from build123d import *

# Parameters (mm, degrees)
ESQUISSE1_W                                        = 11
ESQUISSE1_H                                        = 6
BOSS_EXTRU_1_DEPTH                                 = 22
DIAM_TRE_DU_PER_AGE_7_1_7_1_1_D                    = 7.1
DIAM_TRE_DU_PER_AGE_7_1_7_1_1_DEPTH                = 6
DIAM_TRE_DU_PER_AGE_8_5_8_5_1_D                    = 8.5
CHAMBRAGE_POUR_VIS_T_TE_HEXAGONALE_M21_D           = 2.5
CHAMBRAGE_POUR_VIS_T_TE_HEXAGONALE_M21_CBORE_D     = 4
CHAMBRAGE_POUR_VIS_T_TE_HEXAGONALE_M21_CBORE_DEPTH = 4.5
DIAM_TRE_DU_PER_AGE_8_0_8_1_D                      = 8
DIAM_TRE_DU_PER_AGE_8_0_8_1_DEPTH                  = 2
DIAM_TRE_DU_PER_AGE_8_0_8_1_TIP                    = 4
CHANFREIN1_SIZE                                    = 9
CHANFREIN1_SIZE2                                   = 4.785384885
ENL_V_MAT_EXTRU_1_DEPTH                            = 10


with BuildPart() as part:
    # Esquisse1 → Révolution1 (revolve)
    with BuildSketch(Plane(origin=(0, 0, 0), x_dir=(-1, 0, 0), z_dir=(0, 0, -1)), mode=Mode.PRIVATE) as r_volution1_sk:
        with Locations((-5.5, 3)):
            Rectangle(ESQUISSE1_W, ESQUISSE1_H)
    revolve(r_volution1_sk.sketch.rotate(Axis((0, 0, 0), (0, 1, 0)), 270), axis=Axis((0, 0, 0), (0, 1, 0)))

    # Esquisse2 → Boss.-Extru.1 (add)
    with BuildSketch(Plane(origin=(0, 6, 0), x_dir=(-1, 0, 0), z_dir=(0, 1, 0))):
        Polygon((-9.95156463, 2.63938656), (-3.016441782, 9.843834567), (10.088792211, -2.771484138), (3.016441782, -9.843834567), align=None)
    extrude(amount=BOSS_EXTRU_1_DEPTH)

    # Diamètre du perçage Ø7.1 (7.1)1
    with Locations(Plane(origin=(0, 28, 0), x_dir=(1, 0, 0), z_dir=(0, 1, 0))):
        with Locations((0, 0)):
            Hole(DIAM_TRE_DU_PER_AGE_7_1_7_1_1_D / 2, depth=DIAM_TRE_DU_PER_AGE_7_1_7_1_1_DEPTH)

    # Diamètre du perçage Ø8.5 (8.5)1 (through all)
    with Locations(Plane(origin=(-3.467561424, 0, 3.602224003), x_dir=(0.7204448006982934, 0, 0.6935122847843406), z_dir=(-0.6935122847843406, 0, 0.7204448006982934))):
        with Locations((-0.19047619, 17)):
            Hole(DIAM_TRE_DU_PER_AGE_8_5_8_5_1_D / 2)

    # Chambrage pour vis à tête hexagonale M21 (through all)
    with Locations(Plane(origin=(0, 6, 0), x_dir=(1, 0, 0), z_dir=(0, 1, 0))):
        with Locations((5.656854249, 5.656854249), (-5.656854249, -5.656854249)):
            CounterBoreHole(CHAMBRAGE_POUR_VIS_T_TE_HEXAGONALE_M21_D / 2, CHAMBRAGE_POUR_VIS_T_TE_HEXAGONALE_M21_CBORE_D / 2, CHAMBRAGE_POUR_VIS_T_TE_HEXAGONALE_M21_CBORE_DEPTH)

    # Diamètre du perçage Ø8.0 (8)1
    with Locations(Plane(origin=(0, 0, 0), x_dir=(-1, 0, 0), z_dir=(0, -1, 0))):
        with Locations((0, 0)):
            Hole(DIAM_TRE_DU_PER_AGE_8_0_8_1_D / 2, depth=DIAM_TRE_DU_PER_AGE_8_0_8_1_DEPTH)
            with Locations((0, 0, -(DIAM_TRE_DU_PER_AGE_8_0_8_1_DEPTH + DIAM_TRE_DU_PER_AGE_8_0_8_1_TIP / 2))):  # 90° drill point
                Cone(0, DIAM_TRE_DU_PER_AGE_8_0_8_1_D / 2, DIAM_TRE_DU_PER_AGE_8_0_8_1_TIP, mode=Mode.SUBTRACT)

    # Chanfrein1
    chanfrein1_edges = [part.edges().sort_by_distance(p)[0] for p in [
        (-6.552616997, 28, -6.307659352),
    ]]
    chanfrein1_side = [part.faces().sort_by_distance(p)[0] for p in [
        (-6.552616997, 17, -6.307659352),
    ]]
    chamfer(chanfrein1_edges, length=CHANFREIN1_SIZE, length2=CHANFREIN1_SIZE2, reference=chanfrein1_side[0])

    # Esquisse11 → Enlèv. mat.-Extru.1 (cut)
    with BuildSketch(Plane(origin=(0, 6, 0), x_dir=(1, 0, 0), z_dir=(0, 1, 0))):
        Polygon((1.20429729, -11.726353602), (11.620583405, -0.905551522), (15.545873169, -4.684101481), (5.129587053, -15.504903562), align=None)
        Polygon((0.545569668, 13.405846017), (-12.47793973, 0.382336619), (-16.03995118, 3.944348069), (-3.016441782, 16.967857467), align=None)
    extrude(amount=-ENL_V_MAT_EXTRU_1_DEPTH, mode=Mode.SUBTRACT)


solid = part.part
Could you check a few things on this model? Use its own coordinates, in mm. A direction names the side the tool comes from. Coordinates: 2 decimals unless noted, no trailing zeros. Loops run counter-clockwise (first coordinate to the right, second up) from the corner with the lowest first, then second, coordinate; pieces in that order, holes last. Notation, with made-up numbers: (31.5, 80.25) -> (49.5, 80.25) arc R18 cw to (49.5, 107.25) -> close; hole circle Ø3 at (44, 5.5). An arc over 180 degrees is marked (long way). Answer in a Markdown table with one row per item.
(1) Imagine slicing it at C-C (y = 16.25). List the corners of the cut face in (x, z) for me.
Results found:
| item | result |
|---|---|
| outline | (-10.09, -2.77) -> (-3.02, -9.84) -> (0.32, -6.64) -> (-6.62, 0.57) -> close; (-0.59, 6.37) -> (6.34, -0.83) -> (9.95, 2.64) -> (3.02, 9.84) -> close |
(2) Imagine slicing it at B-B (x = 8.5). List the corners of the cut face in (y, z) for me, plus the area to 3 significant figures.
Results found:
| item | result |
|---|---|
| outline | (0, -6.98) -> (6, -6.98) -> (6, 1.24) -> (28, 1.24) -> (28, 4.15) -> (0, 4.15) -> close |
| area | 131 mm^2 |
(3) For faces 4 (the face through (-0.867, 1.014, 3.905)), 5 (the face through (-0.53, 14.4, 6.43)), 6 (the face through (6, 1.5, -4)), which set-ups out of +Z, -Z, +X, -X, +Y, -Y let a thin tool reach every point of the face, with its end or its side?
Results found:
| item | result |
|---|---|
| face 4 | -Y |
| face 5 | +Z, -X, +Y |
| face 6 | +Y |
(4) Thinking about a two-plate mould opening in Z: for faces 1 (the face through (-7.131, 3.782, 4.305)), 2 (the face through (-6.49, 9.37, -6.37)), 3 (the face through (-3, 6, 6)), which applies, released by +Z, released by -Z, zero draft, split by the parting line, or undercut?
Results found:
| item | result |
|---|---|
| face 1 | undercut |
| face 2 | released by -Z |
| face 3 | zero draft |
(5) Imagine slicing it at A-A (y = 3.5). List the corners of the cut face in (x, z) for me, plus the area to 3 significant figures.
Results found:
| item | result |
|---|---|
| outline | (-10.81, -2.05) -> (-2.05, -10.81) arc R11 ccw to (10.87, 1.69) -> (2.1, 10.8) arc R11 ccw to start; hole circle Ø4 at (-5.66, 5.66); hole circle Ø5 at (0, 0); hole circle Ø4 at (5.66, -5.66) |
| area | 302 mm^2 |
(6) Imagine slicing it at D-D (y = 26.75). List the corners of the cut face in (x, z) for me, plus the area to 3 significant figures.
Results found:
| item | result |
|---|---|
| outline | (-7.12, 0.09) -> (-0.05, -6.99) -> (9.95, 2.64) -> (3.02, 9.84) -> close; hole circle Ø7.1 at (0, 0) |
| area | 100 mm^2 |
(7) If I drill on probe 1 along Z at (x, y) = (0, 0.55); probe 2 along Y at (x, z) = (-1.5, -4.5); probe 3 along Y at (x, z) = (-5.75, 9.25), over which ranges is the centre line in solid material (lowest first)?
Results found:
| item | result |
|---|---|
| probe 1 | z = -11 to -4, 4 to 11 |
| probe 2 | y = 0 to 15.59, 18.41 to 28 |
| probe 3 | y = 0 to 6 |
(8) Will these pins go through, and if not, where does the flat tip stop? pin 1 Ø1.5 at (x, z) = (2.5, -3) entering from -Y; pin 2 Ø3 at (y, z) = (15, -4.5) entering from +X; pin 3 Ø3 at (x, z) = (-6.5, 5) entering from +Y; pin 4 Ø2 at (y, z) = (16.5, 9) entering from -X.
Results found:
| item | result |
|---|---|
| pin 1 | stops at y = 0 |
| pin 2 | stops at x = 1.07 |
| pin 3 | stops at y = 6 |
| pin 4 | stops at x = 1.1 |
